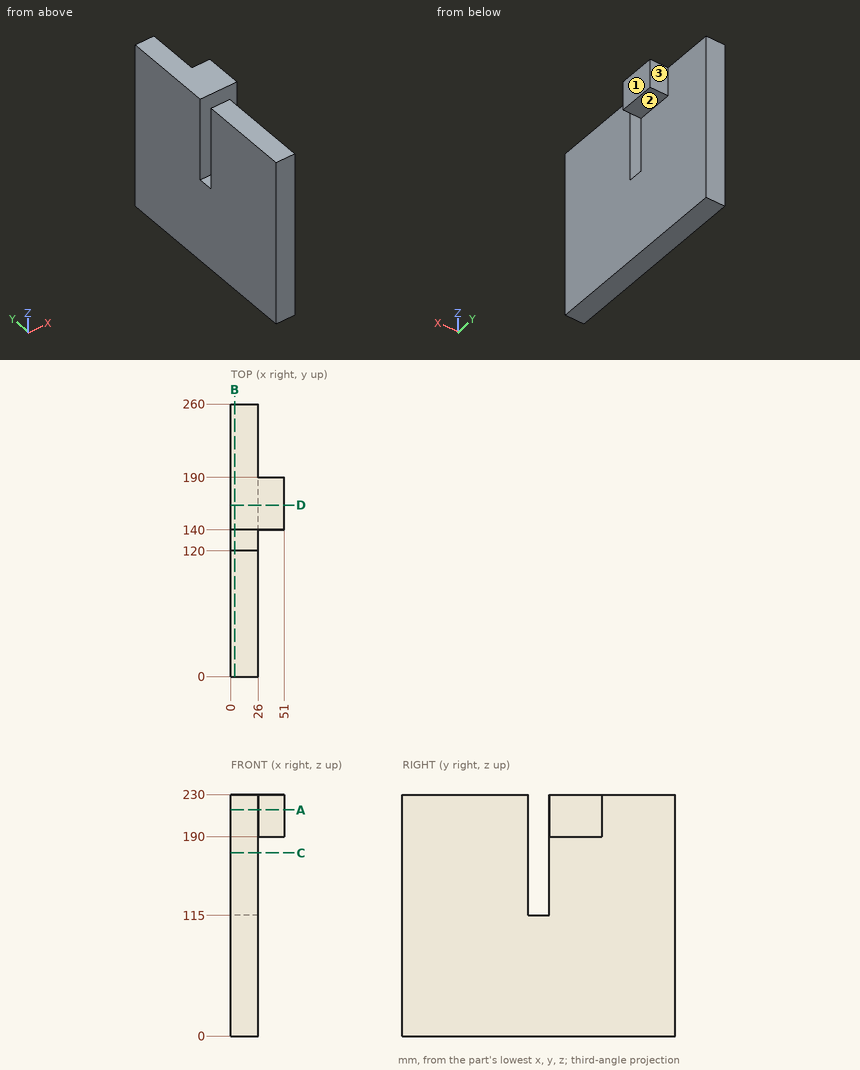
Source: three-view drawing plus pictorial views. Frame: mm from the lowest corner of the part. A direction names the side the tool comes from. Coordinates: 2 decimals unless noted, no trailing zeros. Loops run counter-clockwise (first coordinate to the right, second up) from the corner with the lowest first, then second, coordinate; pieces in that order, holes last. Notation, with made-up numbers: (52, -25) -> (62, -25) arc R16 ccw to (62, -10) -> close; hole circle Ø5 at (25, 20). An arc over 180 degrees is marked (long way). Answer in a Markdown table with one row per item. Add a question column.
Q1. Section B-B on x = 3.5. Return the cut outline in (y, z).
Q2. Contact query for flat-ended pins moving along their axis: pin 1 Ø7.5 at (x, z) = (34, 210) entering from +Y; pin 2 Ø6 at (x, y) = (8.5, 132.5) entering from +Z; pin 3 Ø8 at (x, z) = (32.5, 111.5) entering from +Y; pin 4 Ø3 at (y, z) = (38.5, 92) entering from +X. Output: stop coordinate, or through.
Q3. Ray query, line 1 along Y through (x, z) = (7, 117.5); line 2 along X through (y, z) = (93.5, 18); line 3 along Z through (x, y) = (39.5, 167). Return the intervals inside material, ascending.
Q4. Section A-A on z = 215.5. Return the cut outline in (x, y).
Q5. Section C-C on z = 174.5. Return the cut outline in (x, y), and give its area (3 significant figures).
Q6. Reachability of the marked faces 1, 2 and 3 from +Z, -Z, +X, -X, +Y, -Y: full face, straight path, thin tool, end or side. Return the list, or none.
Q7. Section D-D on y = 163.5. Return the cut outline in (x, z).
Computed values:
| question | item | result |
|---|---|---|
| 1 | outline | (0, 0) -> (260, 0) -> (260, 230) -> (140, 230) -> (140, 115) -> (120, 115) -> (120, 230) -> (0, 230) -> close |
| 2 | pin 1 | stops at y = 190 |
| 2 | pin 2 | stops at z = 115 |
| 2 | pin 3 | passes through |
| 2 | pin 4 | stops at x = 26 |
| 3 | line 1 | y = 0 to 120, 140 to 260 |
| 3 | line 2 | x = 0 to 26 |
| 3 | line 3 | z = 190 to 230 |
| 4 | outline | (0, 0) -> (26, 0) -> (26, 120) -> (0, 120) -> close; (0, 140) -> (51, 140) -> (51, 190) -> (26, 190) -> (26, 260) -> (0, 260) -> close |
| 5 | outline | (0, 0) -> (26, 0) -> (26, 120) -> (0, 120) -> close; (0, 140) -> (26, 140) -> (26, 260) -> (0, 260) -> close |
| 5 | area | 6,240 mm^2 |
| 6 | face 1 | +Z, -Z, +X, +Y, -Y |
| 6 | face 2 | -Z, +X, +Y, -Y |
| 6 | face 3 | +Z, -Z, +X, +Y |
| 7 | outline | (0, 0) -> (26, 0) -> (26, 190) -> (51, 190) -> (51, 230) -> (0, 230) -> close |
